Here's the drawing with two shaded views (mm, measured from the low corner). I have some questions. Coordinates: 2 decimals unless noted, no trailing zeros. Order: outer loops, then holes, each group sorted by start corner. A loop starts at its lowest first (then second) coordinate and runs counter-clockwise, first axis right, second up. Notation, with made-up numbers: (26.25, -22) - (61.25, -22) arc R24 cw to (61.25, 3) - close; hole circle Ø6 at (77, -40). An arc over 180 degrees is marked (long way). One line per item, written item: value. Start each with the question number.
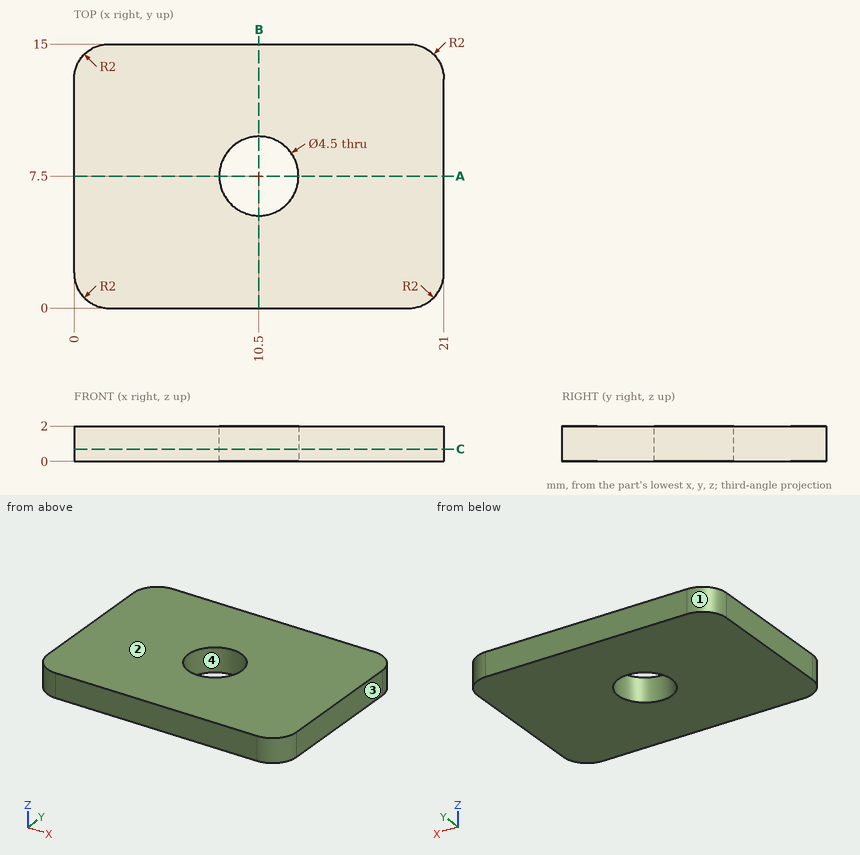
Q1. I want a section at A-A on y = 7.5. Please give me the cut outline in (x, z).
Q2. I'm going to push a flat-ended pin straight in: pin 1 (8 mm diameter, centred on x = 9.5, y = 3, fed in from -Z). Where does the tip first touch, or does it pass through?
Q3. I want a section at B-B on x = 10.5. Please give me the cut outline in (y, z), then the cut area to 3 significant figures.
Q4. If I drill on L1, parallel to Y at x = 10.5, z = 1; L2, parallel to Y at x = 12.5, z = 1.45; L3, parallel to X at y = 6.5, z = 0.3, over which ranges is the centre line in solid material (lowest first)?
Q5. I want a section at C-C on z = 0.7. Please give me the cut outline in (x, y).
Q6. We'd pull the mould along X, two halves only. Please class the marked faces 1, 2, 3 and 4: +X half, -X half, draft (parallel to the pull), parting line (faces both ways), or undercut.
Values follow:
1. outline: (0, 0) - (8.25, 0) - (8.25, 2) - (0, 2) - close; (12.75, 0) - (21, 0) - (21, 2) - (12.75, 2) - close
2. pin 1: stops at z = 0
3. outline: (0, 0) - (5.25, 0) - (5.25, 2) - (0, 2) - close; (9.75, 0) - (15, 0) - (15, 2) - (9.75, 2) - close
3. area: 21.0 mm^2
4. L1: y = 0 to 5.25, 9.75 to 15
4. L2: y = 0 to 6.47, 8.53 to 15
4. L3: x = 0 to 8.48, 12.52 to 21
5. outline: (0, 2) arc R2 ccw to (2, 0) - (19, 0) arc R2 ccw to (21, 2) - (21, 13) arc R2 ccw to (19, 15) - (2, 15) arc R2 ccw to (0, 13) - close; hole circle Ø4.5 at (10.5, 7.5)
6. face 1: -X half
6. face 2: draft
6. face 3: +X half
6. face 4: undercut
